from build123d import *

# Parameters (mm, degrees)
CROQUIS1_R              = 6
CROQUIS1_R_2            = 3
SALIENTE_EXTRUIR1_DEPTH = 14
CORTAR_EXTRUIR1_START   = -3
CROQUIS3_R              = 15
CORTAR_EXTRUIR1_DEPTH   = 8
REDONDEO1_R             = 4


with BuildPart() as part:
    # Croquis1 → Saliente-Extruir1 (new body)
    # profile 1 of 5: a face of its own
    with BuildSketch(Plane.XY):
        with BuildLine():
            ThreePointArc((-23.725422134, 109.136941816), (-3.343361872, 121.724461131), (4.62711067, 144.315290918))
            ThreePointArc((4.62711067, 144.315290918), (-8.782059543, 172.344818376), (-39.020356526, 179.493640019))
            ThreePointArc((-39.020356526, 179.493640019), (-33.980640362, 178.302169745), (-31.74577866, 173.630581835))
            ThreePointArc((-31.74577866, 173.630581835), (-33.07419075, 169.865443538), (-36.471200794, 167.767523652))
            ThreePointArc((-36.471200794, 167.767523652), (-7.920656596, 149.413602382), (-26.274577866, 120.863058184))
            ThreePointArc((-26.274577866, 120.863058184), (-21.234861702, 119.67158791), (-19, 115))
            ThreePointArc((-19, 115), (-20.32841209, 111.234861702), (-23.725422134, 109.136941816))
        make_face()
    # profile 2 of 5: a face of its own
    with BuildSketch(Plane.XY):
        with Locations((-37.74577866, 173.630581835)):
            Circle(CROQUIS1_R)
        with Locations((-37.74577866, 173.630581835)):
            Circle(CROQUIS1_R_2, mode=Mode.SUBTRACT)
    # profile 3 of 5: a face of its own
    with BuildSketch(Plane.XY):
        with Locations((-25, 115)):
            Circle(CROQUIS1_R)
        with Locations((-25, 115)):
            Circle(CROQUIS1_R_2, mode=Mode.SUBTRACT)
    # profile 4 of 5: a face of its own
    with BuildSketch(Plane.XY):
        with BuildLine():
            Line((5.998914104, 0.114147164), (4.62711067, 144.315290918))
            ThreePointArc((4.62711067, 144.315290918), (-3.343361872, 121.724461131), (-23.725422134, 109.136941816))
            Line((-23.725422134, 109.136941816), (-16, 109.136941816))
            ThreePointArc((-16, 109.136941816), (-8.928932188, 106.208009628), (-6, 99.136941816))
            Line((-6, 99.136941816), (-6, 0))
            ThreePointArc((-6, 0), (-0.057076164, 5.99972852), (5.998914104, 0.114147164))
        make_face()
    # profile 5 of 5: a face of its own
    with BuildSketch(Plane.XY):
        with BuildLine():
            Line((6, 0), (5.998914104, 0.114147164))
            ThreePointArc((5.998914104, 0.114147164), (-0.057076164, 5.99972852), (-6, 0))
            ThreePointArc((-6, 0), (0, -6), (6, 0))
        make_face()
        Circle(CROQUIS1_R_2, mode=Mode.SUBTRACT)
    extrude(amount=SALIENTE_EXTRUIR1_DEPTH)

    # Croquis3 → Cortar-Extruir1 (cut)
    with BuildSketch(Plane.XY.offset(14).offset(CORTAR_EXTRUIR1_START)):
        with Locations((-37.74577866, 173.630581835)):
            Circle(CROQUIS3_R)
    extrude(amount=-CORTAR_EXTRUIR1_DEPTH, mode=Mode.SUBTRACT)

    # Redondeo1
    redondeo1_edges = [part.edges().sort_by_distance(p)[0] for p in [
        (-22.748314626, 173.3547693, 11),
        (-22.748314626, 173.3547693, 3),
    ]]
    fillet(redondeo1_edges, radius=REDONDEO1_R - 0.0001)  # a hair under: the kernel refuses the full size


solid = part.part
Could you check a few things on this model? Use its own coordinates, in mm. A direction names the side the tool comes from. Give positions to 0.01 mm unless a question says otherwise; leave off trailing zeros. Order: outer loops, then holes, each group sorted by start corner. A loop starts at its lowest first (then second) coordinate and runs counter-clockwise, first axis right, second up. Notation, with made-up numbers: (87.25, 76) - (141.25, 76) arc R21 cw to (141.25, 84) - close; hole circle Ø7 at (-8, 85). An arc over 180 degrees is marked (long way). Return JSON: item names as keys, results as strings. Group by question number.
Q1. Please list where these lines run through material, in increasing order: line 1 along Y through (x, z) = (-24.5, 2.75); line 2 along Y through (x, z) = (-25, 11.25); line 3 along Z through (x, y) = (-40, 168.5). Write a range as [from, to].
Q2. Suppose I cut it at B-B, the plane y = 115. Please give me the cut outline in (x, z), and give its area (3 significant figures).
Q3. Which directions (+Z, -Z, +X, -X, +Y, -Y) give clear straight access to the entire face, cutting with the end or side of a thin tool? Please do faces 4 (the face through (-3, 0, 7)), 5 (the face through (-6, 50, 7)).
Q4. Suppose I cut it at D-D, the plane y = 68. Please give me the cut outline in (x, z).
Q5. Will these pins go through, and if not, where does the flat tip stop? pin 1 Ø10 at (x, y) = (-39.5, 173.5) entering from +Z; pin 2 Ø8 at (y, z) = (124.5, 5) entering from +X; pin 3 Ø4 at (y, z) = (30, 8) entering from -X; pin 4 Ø6 at (x, z) = (-21.5, 5) entering from -Y.
Q6. Thinking about a two-plate mould opening in Y: for faces 1 (the face through (-6, 101, 14)), 2 (the face through (-20, 109.137, 7)), 3 (the face through (-36.13, 176.16, 12.48)), which applies, pulls with the +Y half, pulls with the -Y half, needs draft (parallel to the pull), parting line crosses it, or undercut?
Q7. Suppose I cut it at A-A, the plane x = 0. Please give me the cut outline in (y, z).
Q8. Suppose I cut it at C-C, the plane z = 4.75. Please give me the cut outline in (x, y), and give its area (3 significant figures).
Resolved:
{
 "1": {"line 1": "y = [109.02, 112.04], [117.96, 121.32], [167.31, 179.65]", "line 2": "y = [109, 112], [118, 121.18], [167.45, 179.75]", "line 3": "z = [0, 3], [11, 14]"},
 "2": {"outline": "(-31, 0) - (-28, 0) - (-28, 14) - (-31, 14) - close; (-22, 0) - (4.91, 0) - (4.91, 14) - (-22, 14) - close", "area": "419 mm2"},
 "3": {"face 4": "+Z, -Z", "face 5": "+Z, -Z, -X, -Y"},
 "4": {"outline": "(-6, 0) - (5.35, 0) - (5.35, 14) - (-6, 14) - close"},
 "5": {"pin 1": "stops at z = 14", "pin 2": "stops at x = 4.85", "pin 3": "stops at x = -6", "pin 4": "stops at y = 109.02"},
 "6": {"face 1": "needs draft", "face 2": "pulls with the -Y half", "face 3": "undercut"},
 "7": {"outline": "(-6, 0) - (-3, 0) - (-3, 14) - (-6, 14) - close; (3, 0) - (161.97, 0) - (161.97, 14) - (3, 14) - close"},
 "8": {"outline": "(-26.27, 120.86) arc R6 ccw to (-23.73, 109.14) - (-16, 109.14) arc R10 cw to (-6, 99.14) - (-6, 0) arc R6 ccw to (6, 0) - (4.63, 144.32) arc R36 ccw to (-24.79, 179.71) arc R14.31 cw to (-24.86, 167.41) arc R24 cw to start; hole circle Ø6 at (-25, 115); hole circle Ø6 at (0, 0)", "area": "2,550 mm2"}
}
